Geometry: final body of the model. Coordinates: model frame, mm. Face numbers are marked on the shaded views. A direction names the side the tool comes from. Give positions to 0.01 mm unless a question says otherwise; leave off trailing zeros. Write each loop counter-clockwise with the first axis right and the second up, starting at its lowest first coordinate (ties: lowest second). Pieces come first, ordered by that corner, then holes. Notation, with made-up numbers: (-21.75, 51.5) -> (-7.75, 51.5) arc R30 cw to (-7.75, 77.5) -> close; hole circle Ø9 at (73.25, 69). An arc over 180 degrees is marked (long way). Answer as a JSON object with one key per item and string values. Group by question number.
(1) Section query A-A on z = 0. Output: boundary loops of the cut face in (x, y).
(2) Section query C-C on y = 0. Output: boundary loops of the cut face in (x, z).
(3) Section query D-D on x = 0.95. State how many separate pieces and enclosed holes the cut face has, plus the area to 3 significant figures.
(4) Set-up query: the marked faces 1, 2, 3 and 4. Return all of +Z, -Z, +X, -X, +Y, -Y with unobstructed straight access to the full face (end or side cutting, diameter ignored); none if empty.
(5) Draft query along Z for the marked faces 5, 6, 7 and 8. Return one class per face: +Z half, -Z half, draft (parallel to the pull), parting line (faces both ways), or undercut.
(6) Section query B-B on y = 27. Output: boundary loops of the cut face in (x, z).
(7) Contact query for a flat-ended pin moving along its axis: pin 1 Ø1 at (x, z) = (2.5, 6.5) entering from +Y. Output: stop coordinate, or through.
(8) Material intervals for probe 1 along Y at (x, z) = (1.15, 0); probe 2 along Y at (x, z) = (0.3, 0.5); probe 3 along Z at (x, y) = (2.65, 10.5), sorted ascending.
from build123d import *

# Parameters (mm, degrees)
BASPROSKE_W         = 3
BASPROSKE_H         = 16.5
TOOTHCUT_DEPTH      = 24.526580712
TEETHCUTS_COUNT     = 20
TEETHCUTS_ANGLE     = 342
EXTRUDE_3_DEPTH     = 3
SKETCH_3_R          = 2.5
CUT_EXTRUDE_2_DEPTH = 36.618883333


with BuildPart() as part:
    # BasProSke → Base-Revolve (revolve)
    with BuildSketch(Plane(origin=(0, 0, 0), x_dir=(1, 0, 0), z_dir=(0, 1, 0)), mode=Mode.PRIVATE) as base_revolve_sk:
        with Locations((1.5, 8.25)):
            Rectangle(BASPROSKE_W, BASPROSKE_H)
    revolve(base_revolve_sk.sketch.rotate(Axis((-10, 0, 0), (1, 0, 0)), 180), axis=Axis((-10, 0, 0), (1, 0, 0)))

    # TooCutSke → ToothCut (cut, through all)
    with BuildSketch(Plane(origin=(0, 0, 0), x_dir=(0, 0, -1), z_dir=(1, 0, 0))):
        with BuildLine():
            ThreePointArc((0.74381438, 13.102904875), (0, 13.124), (-0.74381438, 13.102904875))
            ThreePointArc((-0.74381438, 13.102904875), (-1.226473103, 14.852072512), (-2.209965745, 16.376962373))
            ThreePointArc((-2.209965745, 16.376962373), (0, 16.5254), (2.209965745, 16.376962373))
            ThreePointArc((2.209965745, 16.376962373), (1.226473103, 14.852072512), (0.74381438, 13.102904875))
        make_face()
    toothcut = extrude(amount=TOOTHCUT_DEPTH, mode=Mode.SUBTRACT)

    # TeethCuts: ToothCut ×20 about axis
    teethcuts_axis = Axis((-10, 0, 0), (1, 0, 0))
    for i in range(1, TEETHCUTS_COUNT):
        add(toothcut.rotate(teethcuts_axis, i * TEETHCUTS_ANGLE / (TEETHCUTS_COUNT - 1)), mode=Mode.SUBTRACT)

    # 草图2 → 凸台-拉伸3 (add)
    with BuildSketch(Plane.ZY):
        with BuildLine():
            Line((-3.5, 0), (-3.5, 28))
            ThreePointArc((-3.5, 28), (0, 31.5), (3.5, 28))
            Line((3.5, 28), (3.5, 0))
            ThreePointArc((3.5, 0), (0, -3.5), (-3.5, 0))
        make_face()
    extrude(amount=-EXTRUDE_3_DEPTH)

    # 草图3 → 切除-拉伸2 (cut, through all)
    with BuildSketch(Plane.ZY):
        Circle(SKETCH_3_R)
        with Locations((0, 27)):
            Circle(SKETCH_3_R)
    extrude(amount=-CUT_EXTRUDE_2_DEPTH, mode=Mode.SUBTRACT)


solid = part.part
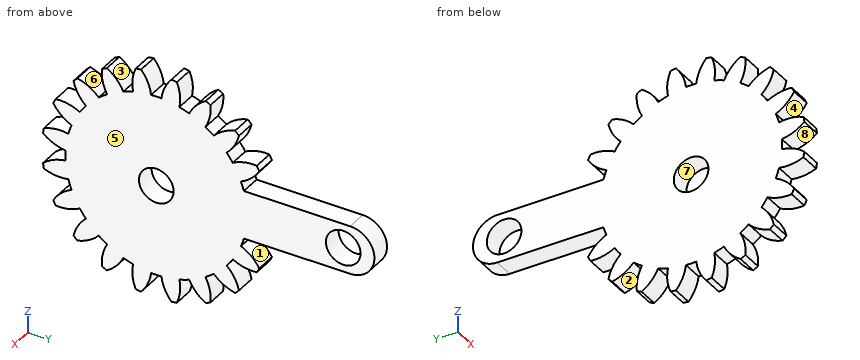
Answer list:
{
 "1": {"outline": "(0, -13.12) -> (3, -13.12) -> (3, -2.5) -> (0, -2.5) -> close; (0, 2.5) -> (3, 2.5) -> (3, 24.5) -> (0, 24.5) -> close; (0, 29.5) -> (3, 29.5) -> (3, 31.5) -> (0, 31.5) -> close"},
 "2": {"outline": "(0, -13.12) -> (3, -13.12) -> (3, -2.5) -> (0, -2.5) -> close; (0, 2.5) -> (3, 2.5) -> (3, 13.12) -> (0, 13.12) -> close"},
 "3": {"separate pieces": "1", "enclosed holes": "2", "area": "753 mm2"},
 "4": {"face 1": "+X, -X, +Y", "face 2": "-Z, +X, -X", "face 3": "+Z, +X, -X", "face 4": "+X, -X, -Y"},
 "5": {"face 5": "draft", "face 6": "+Z half", "face 7": "undercut", "face 8": "undercut"},
 "6": {"outline": "(0, -3.5) -> (3, -3.5) -> (3, -2.5) -> (0, -2.5) -> close; (0, 2.5) -> (3, 2.5) -> (3, 3.5) -> (0, 3.5) -> close"},
 "7": {"pin 1": "y = 14.79"},
 "8": {"probe 1": "-13.12 to -2.5, 2.5 to 24.5, 29.5 to 31.5", "probe 2": "-13.11 to -2.45, 2.45 to 24.55, 29.45 to 31.46", "probe 3": "-11.67 to -8.64, -7.87 to 7.87, 8.64 to 11.67"}
}
